```python
from build123d import *

# Parameters (mm, degrees)
F0_W     = 396
F0_H     = 396
F1_DEPTH = 19
F2_R     = 140.5
F3_DEPTH = 25.4
F4_R     = 2.25
F5_DEPTH = 25.4


with BuildPart() as f1:
    # F0 (on Front) → F1 (new body)
    with BuildSketch(Plane.XZ):
        Rectangle(F0_W, F0_H)
    extrude(amount=F1_DEPTH)

    # F2 (on face) → F3 (cut)
    with BuildSketch(Plane.XZ.offset(19)):
        Circle(F2_R)
    extrude(amount=-F3_DEPTH, mode=Mode.SUBTRACT)

    # F4 (on face) → F5 (cut)
    with BuildSketch(Plane.XZ.offset(19)):
        with Locations((57.670393, 139.228646)):
            Circle(F4_R)
        with Locations((139.228646, 57.670393)):
            Circle(F4_R)
        with Locations((139.228646, -57.670393)):
            Circle(F4_R)
        with Locations((57.670393, -139.228646)):
            Circle(F4_R)
        with Locations((-57.670393, -139.228646)):
            Circle(F4_R)
        with Locations((-139.228646, -57.670393)):
            Circle(F4_R)
        with Locations((-139.228646, 57.670393)):
            Circle(F4_R)
        with Locations((-57.670393, 139.228646)):
            Circle(F4_R)
    extrude(amount=-F5_DEPTH, mode=Mode.SUBTRACT)


solid = f1.part
```
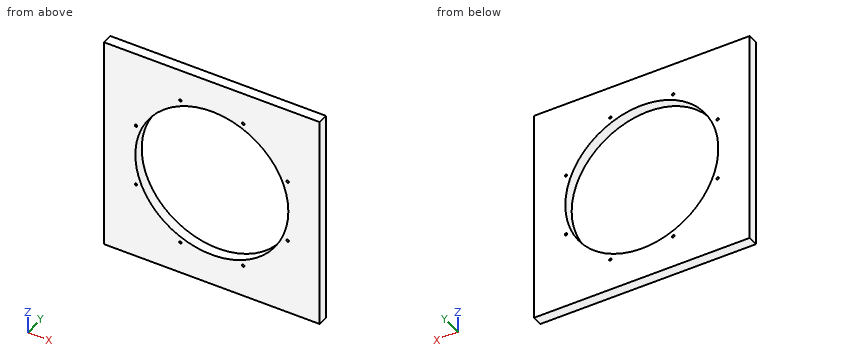
Check sheet for the modelled part. Datum: model origin and axes. Units: mm. Round coordinates to 2 decimals unless told otherwise and drop trailing zeros. Order: outer loops, then holes, each group sorted by start corner. A loop starts at its lowest first (then second) coordinate and runs counter-clockwise, first axis right, second up.
1) Go/stop test with a flat-tipped pin: pin 1 Ø2.5 at (x, z) = (57.67, -139.23) entering from +Y. Record where the tip stops, or that it passes through.
2) Section check C-C (y = -5). Give the number of separate pieces and of enclosed holes in the cut face, and give its area (3 significant figures).
3) Section check B-B (x = 0). Record the boundary of the cut face in (y, z), and give its area (4 significant figures).
4) Scan lines: line 1 (Z direction, x = 0, y = -8.25); line 2 (Z direction, x = -18, y = -5.5); line 3 (X direction, y = -5, z = 80). Record each from-to range of solid material in increasing order.
5) Section check A-A (z = 0). Record the boundary of the cut face in (x, y), and give its area (4 significant figures).
Result:
1. pin 1: passes through
2. separate pieces: 1
2. enclosed holes: 9
2. area: 94,700 mm2
3. outline: (-19, -198) - (0, -198) - (0, -140.5) - (-19, -140.5) - close; (-19, 140.5) - (0, 140.5) - (0, 198) - (-19, 198) - close
3. area: 2,185 mm2
4. line 1: z = -198 to -140.5, 140.5 to 198
4. line 2: z = -198 to -139.34, 139.34 to 198
4. line 3: x = -198 to -115.5, 115.5 to 198
5. outline: (-198, -19) - (-140.5, -19) - (-140.5, 0) - (-198, 0) - close; (140.5, -19) - (198, -19) - (198, 0) - (140.5, 0) - close
5. area: 2,185 mm2
